Input: part model. Units: mm. Frame: model coordinates. A direction names the side the tool comes from. Coordinates: 2 decimals unless noted, no trailing zeros. Loops run counter-clockwise (first coordinate to the right, second up) from the corner with the lowest first, then second, coordinate; pieces in that order, holes last. Notation, with made-up numbers: (87, -19.75) - (92, -19.75) arc R29 cw to (92, 3.25) - close; hole circle Ø7 at (-19, 17). An arc over 180 degrees is marked (long way). Write item = value, one per line. Start each with the question number.
from build123d import *

# Parameters (mm, degrees)
SKETCH2_R               = 16
BOSS_EXTRUDE1_DEPTH     = 82.25
CUT_EXTRUDE1_DEPTH      = 97.457244414
CUT_EXTRUDE1_DEPTH_BACK = 97.457244414
SKETCH3_W               = 152.01959988
SKETCH3_H               = 124.433031562
CUT_EXTRUDE2_DEPTH      = 1.4
CHAMFER2_SIZE           = 1
CHAMFER3_SIZE           = 1
CUT_EXTRUDE3_DEPTH      = 71
CHAMFER4_SIZE           = 1
CUT_EXTRUDE4_DEPTH      = 1.2
SKETCH8_R               = 2.75
CUT_EXTRUDE5_DEPTH      = 87.332400234
CUT_EXTRUDE7_DEPTH      = 5
CHAMFER5_SIZE           = 0.5
CUT_EXTRUDE8_DEPTH      = 88.459952722
SKETCH12_R              = 1.8
CUT_EXTRUDE9_DEPTH      = 4
CUT_EXTRUDE10_START     = -4
SKETCH13_R              = 1.8
CUT_EXTRUDE10_DEPTH     = 4
SKETCH14_W              = 4.1
SKETCH14_H              = 1.25
CUT_EXTRUDE11_DEPTH     = 87.894692785


with BuildPart() as part:
    # Sketch1 → Revolve1 (revolve)
    with BuildSketch(Plane(origin=(0, 0, 0), x_dir=(1, 0, 0), z_dir=(0, 1, 0))):
        Polygon((0, 0), (16.125, 0), (16.125, -71), (19.65, -71), (19.65, 68), (24.95, 68), (24.95, 73), (28.1, 73), (28.1, 68), (42, 68), (42, 76), (16.65, 76), (16.65, 18.004366875), (12.193967069, 18.004366875), (12.193967069, 24.882682167), (0, 24.882682167), align=None)
    revolve(axis=Axis((0, 0, 39.840023079), (0, 0, -1)))

    # Sketch2 → Boss-Extrude1 (add)
    with BuildSketch(Plane.XY.offset(71)):
        Polygon((0, 22.762034363), (-19.7125, 11.381017181), (-19.7125, -11.381017181), (0, -22.762034363), (19.7125, -11.381017181), (19.7125, 11.381017181), align=None)
        Circle(SKETCH2_R, mode=Mode.SUBTRACT)
    extrude(amount=-BOSS_EXTRUDE1_DEPTH)

    # Sketch3 → Cut-Extrude1 (cut, two sides: drawn at the far end of the back side and taken through both)
    with BuildSketch(Plane(origin=(0, 0, 0), x_dir=(1, 0, 0), z_dir=(0, 1, 0)).offset(-CUT_EXTRUDE1_DEPTH_BACK)):
        with Locations((6.162956752, 73.466515781)):
            Rectangle(SKETCH3_W, SKETCH3_H)
    extrude(amount=CUT_EXTRUDE1_DEPTH + CUT_EXTRUDE1_DEPTH_BACK, mode=Mode.SUBTRACT)

    # Sketch4 → Cut-Extrude2 (cut)
    with BuildSketch(Plane(origin=(-9.85625, 17.071525772, 0), x_dir=(0.8660254037844386, 0.5000000000000003, 0), z_dir=(-0.5000000000000002, 0.8660254037844385, 0))):
        Polygon((-8.6, 10.2), (4.6, 10.2), (4.6, 5.2), (1.6, 5.2), (1.6, -65), (4.6, -65), (4.6, -70), (-8.6, -70), align=None)
    extrude(amount=-CUT_EXTRUDE2_DEPTH, mode=Mode.SUBTRACT)

    # Chamfer2
    chamfer2_edges = [part.edges().sort_by_distance(p)[0] for p in [
        (0, 22.762034363, 29.875),
        (19.7125, 11.381017181, 29.875),
        (19.7125, -11.381017181, 29.875),
        (0, -22.762034363, 29.875),
        (-19.7125, -11.381017181, 29.875),
        (-19.7125, 11.381017181, 29.875),
    ]]
    chamfer(chamfer2_edges, length=CHAMFER2_SIZE)

    # Chamfer3
    chamfer3_edges = [part.edges().sort_by_distance(p)[0] for p in [
        (-16, 0, 71),
    ]]
    chamfer(chamfer3_edges, length=CHAMFER3_SIZE)

    # Sketch5 → Cut-Extrude3 (cut)
    with BuildSketch(Plane.XY.offset(71)):
        with BuildLine():
            Line((-17, 9.814954576), (-15.92887426, -1.50697207))
            ThreePointArc((-15.92887426, -1.50697207), (-8, 13.85640646), (9.269513225, 13.041323728))
            Line((9.269513225, 13.041323728), (0, 19.629909152))
            Line((0, 19.629909152), (-17, 9.814954576))
        make_face()
        with BuildLine():
            Line((0, -19.629909152), (17, -9.814954576))
            Line((17, -9.814954576), (15.92887426, 1.50697207))
            ThreePointArc((15.92887426, 1.50697207), (8, -13.856406461), (-9.269513225, -13.041323728))
            Line((-9.269513225, -13.041323728), (0, -19.629909152))
        make_face()
    extrude(amount=-CUT_EXTRUDE3_DEPTH, mode=Mode.SUBTRACT)

    # Chamfer4
    chamfer4_edges = [part.edges().sort_by_distance(p)[0] for p in [
        (0, -19.629909152, 35.5),
        (17, -9.814954576, 35.5),
        (0, 19.629909152, 35.5),
        (-17, 9.814954576, 35.5),
    ]]
    chamfer(chamfer4_edges, length=CHAMFER4_SIZE)

    # Sketch6 → Cut-Extrude4 (cut)
    with BuildSketch(Plane(origin=(0, 0, -11.25), x_dir=(-1, 0, 0), z_dir=(0, 0, -1))):
        Polygon((-7.216878365, 12.5), (-14.43375673, 0), (-7.216878365, -12.5), (7.216878365, -12.5), (14.43375673, 0), (7.216878365, 12.5), align=None)
    extrude(amount=-CUT_EXTRUDE4_DEPTH, mode=Mode.SUBTRACT)

    # Sketch8 → Cut-Extrude5 (cut, through all)
    with BuildSketch(Plane(origin=(0, 0, -10.05), x_dir=(-1, 0, 0), z_dir=(0, 0, -1))):
        Circle(SKETCH8_R)
    extrude(amount=-CUT_EXTRUDE5_DEPTH, mode=Mode.SUBTRACT)

    # Sketch10 → Cut-Extrude7 (cut)
    with BuildSketch(Plane.XY):
        with BuildLine():
            Line((2.5, 10), (-2.5, 10))
            Line((-2.5, 10), (-2.5, 7.071067812))
            ThreePointArc((-2.5, 7.071067812), (0, -7.5), (2.5, 7.071067812))
            Line((2.5, 7.071067812), (2.5, 10))
        make_face()
    extrude(amount=-CUT_EXTRUDE7_DEPTH, mode=Mode.SUBTRACT)

    # Chamfer5
    chamfer5_edges = [part.edges().sort_by_distance(p)[0] for p in [
        (0, -7.5, 0),
        (2.5, 8.535533906, 0),
        (0, 10, 0),
        (-2.5, 8.535533906, 0),
    ]]
    chamfer(chamfer5_edges, length=CHAMFER5_SIZE)

    # Sketch11 → Cut-Extrude8 (cut, through all)
    with BuildSketch(Plane.XY.offset(71)):
        Polygon((19.7125, 11.381017181), (16.660566959, 13.143051544), (19.7125, 7.856948456), align=None)
        Polygon((-16.660566959, -13.143051544), (-19.7125, -11.381017181), (-19.7125, -7.856948456), align=None)
    extrude(amount=-CUT_EXTRUDE8_DEPTH, mode=Mode.SUBTRACT)

    # Sketch12 → Cut-Extrude9 (cut)
    with BuildSketch(Plane(origin=(-18.186533479, -10.5, 0), x_dir=(0, 0, 1), z_dir=(-0.8660254037844382, -0.500000000000001, 0))):
        with Locations(Location((48, 0, 0), (0, 0, 270))):
            Circle(SKETCH12_R)
    extrude(amount=-CUT_EXTRUDE9_DEPTH, mode=Mode.SUBTRACT)

    # Sketch13 → Cut-Extrude10 (cut)
    with BuildSketch(Plane(origin=(18.186533479, 10.5, 0), x_dir=(0, 0, -1), z_dir=(0.8660254037844387, 0.4999999999999999, 0)).offset(CUT_EXTRUDE10_START)):
        with Locations(Location((-48, 0, 0), (0, 0, 270))):
            Circle(SKETCH13_R)
    extrude(amount=CUT_EXTRUDE10_DEPTH, mode=Mode.SUBTRACT)

    # Sketch14 → Cut-Extrude11 (cut, through all)
    with BuildSketch(Plane(origin=(18.186533479, 10.5, 0), x_dir=(0, 0, -1), z_dir=(0.8660254037844387, 0.4999999999999999, 0))):
        with Locations((-63.2, 0)):
            Rectangle(SKETCH14_W, SKETCH14_H)
    extrude(amount=-CUT_EXTRUDE11_DEPTH, mode=Mode.SUBTRACT)


solid = part.part
Item 1: Cut plane A-A on z = 55. Return loops of the section in (x, y), plus the area to 3 significant figures.
Item 2: Pull-direction query (Y, two-part tool) for faces 1 (the flat face through (14.71, 8.52, 47.97)), 2 (the flat face through (0.04, -19.09, 36)), 3 (the flat face through (-8.87, -17.64, 30.45)), 4 (the flat face through (18.165, 10.537, 30.451)); classes: pulls with the +Y half, pulls with the -Y half, needs draft (parallel to the pull), parting line crosses it, or undercut.
Item 3: Cut plane B-B on x = 0. Return loops of the section in (y, z).
Item 4: Ray query, line 1 (X direction, y = 0, z = -1.8); line 2 (Y direction, x = 0, z = -1.7); line 3 (X direction, y = -8, z = 55). Return the intervals inside material, ascending.
Item 5: Pin query (flat end, axial travel): pin 1 (12 mm diameter, centred on x = 6.5, y = 4.5, fed in from +Z); pin 2 (12 mm diameter, centred on x = 0, y = 0, fed in from -Z); pin 3 (1 mm diameter, centred on x = -14, y = -16, fed in from +Z); pin 4 (1.5 mm diameter, centred on y = 8.5, z = -2.5, fed in from +X). Return the tip coordinate at first contact, or that it passes through.
Item 6: Access query for faces 5 (the flat face through (15.734, 9.806, 63.229)), 6 (the flat face through (-19.712, 1, 30)), 7 (the flat face through (-3, 0, -10.05)), 8 (the flat face through (0, 3, -5)). Directions: +Z, -Z, +X, -X, +Y, -Y. A direction counts if a zero-diameter tool reaches every point of the face in a straight line with its end or side. Return the directions, or none.
Recorded:
q1.outline = (-19.71, -7.86) - (-16.66, -13.14) - (-0.87, -22.26) - (0.87, -22.26) - (18.85, -11.88) - (19.71, -10.38) - (19.71, 7.86) - (16.66, 13.14) - (0.87, 22.26) - (-0.87, 22.26) - (-8.47, 17.87) - (-7.77, 16.66) - (-16.6, 11.56) - (-17.3, 12.77) - (-18.85, 11.88) - (-19.71, 10.38) - close; hole (-16.91, 8.82) - (-15.93, -1.51) arc R16 ccw to (-9.27, -13.04) - (-0.82, -19.05) - (0.87, -19.13) - (16.13, -10.31) - (16.91, -8.82) - (15.93, 1.51) arc R16 ccw to (9.27, 13.04) - (0.82, 19.05) - (-0.87, 19.13) - (-16.13, 10.31) - close
q1.area = 404 mm²
q2.face_1 = undercut
q2.face_2 = undercut
q2.face_3 = pulls with the -Y half
q2.face_4 = pulls with the +Y half
q3.outline = (-22.26, -11.25) - (-12.5, -11.25) - (-12.5, -10.05) - (-2.75, -10.05) - (-2.75, -5) - (-7.5, -5) - (-7.5, -0.5) - (-8, 0) - (-19.09, 0) - (-19.09, 71) - (-22.26, 71) - close; (2.75, -10.05) - (12.5, -10.05) - (12.5, -11.25) - (22.26, -11.25) - (22.26, 71) - (19.09, 71) - (19.09, 0) - (10.5, 0) - (10, -0.5) - (10, -5) - (2.75, -5) - close
q4.line_1 = -19.71 to -7.5, 7.5 to 19.71
q4.line_2 = -22.26 to -7.5, 10 to 22.26
q4.line_3 = -19.63 to -13.86, 16.83 to 19.71
q5.pin_1 = 0
q5.pin_2 = -10.05
q5.pin_3 = through
q5.pin_4 = 19.71
q6.face_5 = none
q6.face_6 = +Z, -Z, -X, +Y, -Y
q6.face_7 = -Z
q6.face_8 = +Z
